Autodesk Inventor part; units mm, degrees
ref_plane "YZ Plane" through (0, 0, 0) normal (1, 0, 0) x (0, 1, 0)
ref_plane "XZ Plane" through (0, 0, 0) normal (0, 1, 0) x (-1, 0, 0)
ref_plane "XY Plane" through (0, 0, 0) normal (0, 0, 1) x (1, 0, 0)
sketch "スケッチ1" plane through (0, 0, 0) normal (0, 0, 1) x (1, 0, 0)
  line L0 (0, 0) -> (-1100, 0)
  line L1 (-1100, 0) -> (-1100, 200)
  line L2 (-1100, 200) -> (0, 0)
  dimension "d1" = 1100
  dimension "d2" = 200
extrude "押し出し1" add sketch "スケッチ1" along normal mid plane 600
sketch "スケッチ2" plane through (0, 0, 0) normal (0, 0, 1) x (1, 0, 0)
  line L0 (-1100, 0) -> (0, 0)
  line L1 (0, 0) -> (-1100, 200)
  line L2 (-1100, 200) -> (-1100, 0)
  line L3 (-1100, 200) -> (-1100, 200.1016)
  line L4 (-1100, 200.1016) -> (0.559, 0)
  line L5 (0.559, 0) -> (0, 0)
  dimension "d5" = 0.1
extrude "押し出し2" add sketch "スケッチ2" along normal mid plane 30 contours L1 L3 L4 L5
properties part number "Slope 1"
Model file for the job. Use its own axes, mm. Round coordinates to 2 decimals unless told otherwise and drop trailing zeros. Loops run counter-clockwise (first coordinate to the right, second up) from the corner with the lowest first, then second, coordinate; pieces in that order, holes last.
1. Band-saw the part on C-C, the plane z = -190. List the corners of the cut face in (x, y).
Check values:
outline: (-1100, 0) - (0, 0) - (-1100, 200) - close
2. Wall check: probe 1 along Y at (x, z) = (-961.5, 216.5); probe 2 along Y at (x, z) = (-330, 173). Give the ranges that are in metal, low to high.
Check values:
probe 1: y = 0 to 174.82
probe 2: y = 0 to 60
3. Band-saw the part on A-A, the plane x = -680.5. List the corners of the cut face in (y, z).
Check values:
outline: (0, -300) - (123.73, -300) - (123.73, -15) - (123.83, -15) - (123.83, 15) - (123.73, 15) - (123.73, 300) - (0, 300) - close
4. Band-saw the part on B-B, the plane y = 47. List the corners of the cut face in (x, z), and give its area (3 significant figures).
Check values:
outline: (-1100, -300) - (-258.5, -300) - (-258.5, -15) - (-257.94, -15) - (-257.94, 15) - (-258.5, 15) - (-258.5, 300) - (-1100, 300) - close
area: 505,000 mm2
5. Drop a flat-ended pin along its axis: P1, Ø2, axis at x = -694.5, z = 197.5, coming from the -Y side. Give the stop position or say it passes through.
Check values:
P1: stops at y = 0
